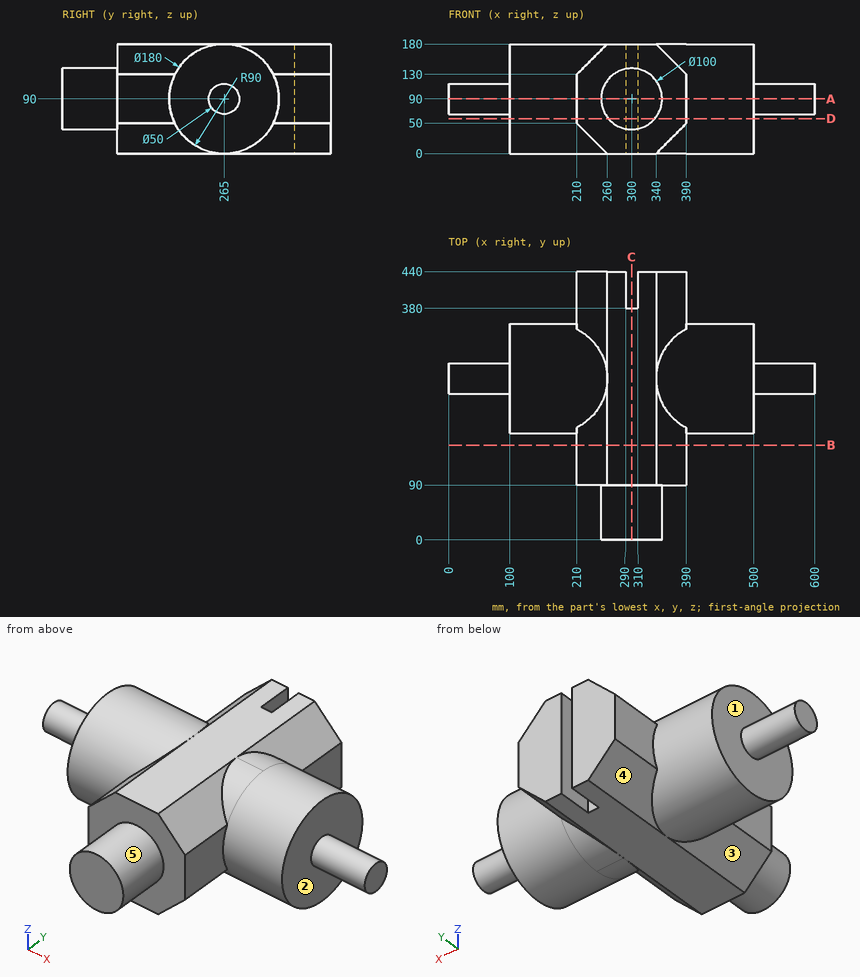
Print and shaded views of the part. All mm, measured from the part's lowest x, y and z. A direction names the side the tool comes from. Round coordinates to 2 decimals unless told otherwise and drop trailing zeros. Order: outer loops, then holes, each group sorted by start corner. A loop starts at its lowest first (then second) coordinate and runs counter-clockwise, first axis right, second up.
Q1. Slice it at C-C (x = 300). Write the cut outline in (y, z), and give its area (3 significant figures).
Q2. Wall check: L1, parallel to X at y = 122, z = 86; L2, parallel to X at y = 213.5, z = 49; L3, parallel to Y at x = 255, z = 12.5. Give the ranges that are in metal, low to high.
Q3. Slice it at A-A (z = 90). Write the cut outline in (x, y), and give its area (3 significant figures).
Q4. Drop flat-ended pins along their axis: pin 1 (12 mm diameter, centred on y = 196.5, z = 161.5, fed in from -X); pin 2 (5 mm diameter, centred on y = 304.5, z = 117, fed in from -X); pin 3 (2 mm diameter, centred on x = 495, y = 321, fed in from +Z). Give the stop position or say it passes through.
Q5. Which spindle directions (+Z, -Z, +X, -X, +Y, -Y) get a long thin tool onto all of the face, cutting with end or side? Do the marked faces 1, 2, 3, 4 and 5. Say none if no direction does.
Q6. Slice it at D-D (z = 57.5). Write the cut outline in (x, y).
Q7. Slice it at B-B (y = 155.5). Write the cut outline in (x, z).
Results below:
1. outline: (0, 40) - (90, 40) - (90, 0) - (380, 0) - (380, 180) - (90, 180) - (90, 140) - (0, 140) - close
1. area: 61,200 mm2
2. L1: x = 210 to 390
2. L2: x = 100 to 500
2. L3: y = 90 to 440
3. outline: (0, 240) - (100, 240) - (100, 175) - (210, 175) - (210, 90) - (250, 90) - (250, 0) - (350, 0) - (350, 90) - (390, 90) - (390, 175) - (500, 175) - (500, 240) - (600, 240) - (600, 290) - (500, 290) - (500, 355) - (390, 355) - (390, 440) - (310, 440) - (310, 380) - (290, 380) - (290, 440) - (210, 440) - (210, 355) - (100, 355) - (100, 290) - (0, 290) - close
3. area: 120,000 mm2
4. pin 1: stops at x = 235.5
4. pin 2: stops at x = 100
4. pin 3: stops at z = 161.24
5. face 1: -X
5. face 2: +X
5. face 3: -Z, -X, -Y
5. face 4: -Z, -X, +Y
5. face 5: -Y
6. outline: (100, 181.07) - (210, 181.07) - (210, 90) - (262, 90) - (262, 0) - (338, 0) - (338, 90) - (390, 90) - (390, 181.07) - (500, 181.07) - (500, 348.93) - (390, 348.93) - (390, 440) - (310, 440) - (310, 380) - (290, 380) - (290, 440) - (210, 440) - (210, 348.93) - (100, 348.93) - close
7. outline: (210, 50) - (260, 0) - (340, 0) - (390, 50) - (390, 130) - (340, 180) - (260, 180) - (210, 130) - close
